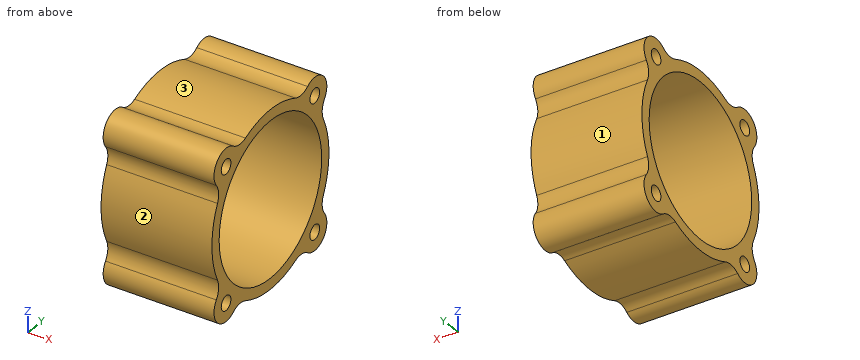
```python
from build123d import *

# Parameters (mm, degrees)
SKETCH_1_R      = 21.25
SKETCH_1_R_2    = 2
EXTRUDE_1_DEPTH = 15.2


with BuildPart() as part:
    # 草图1 → 凸台-拉伸1 (new body, symmetric)
    with BuildSketch(Plane(origin=(0, 0, 0), x_dir=(0, 0, -1), z_dir=(1, 0, 0))):
        with BuildLine():
            ThreePointArc((-15.431825442, 22.419634577), (-21.920310245, 21.920310245), (-22.419634577, 15.431825442))
            ThreePointArc((-22.419634577, 15.431825442), (-21.477282941, 12.955720303), (-21.932357291, 10.345733597))
            ThreePointArc((-21.932357291, 10.345733597), (-24.25, 0), (-21.932357291, -10.345733597))
            ThreePointArc((-21.932357291, -10.345733597), (-21.477282941, -12.955720303), (-22.419634577, -15.431825442))
            ThreePointArc((-22.419634577, -15.431825442), (-21.920310245, -21.920310245), (-15.431825442, -22.419634577))
            ThreePointArc((-15.431825442, -22.419634577), (-12.955720303, -21.477282941), (-10.345733597, -21.932357291))
            ThreePointArc((-10.345733597, -21.932357291), (0, -24.25), (10.345733597, -21.932357291))
            ThreePointArc((10.345733597, -21.932357291), (12.955720303, -21.477282941), (15.431825442, -22.419634577))
            ThreePointArc((15.431825442, -22.419634577), (21.920310245, -21.920310245), (22.419634577, -15.431825442))
            ThreePointArc((22.419634577, -15.431825442), (21.477282941, -12.955720303), (21.932357291, -10.345733597))
            ThreePointArc((21.932357291, -10.345733597), (24.25, 0), (21.932357291, 10.345733597))
            ThreePointArc((21.932357291, 10.345733597), (21.477282941, 12.955720303), (22.419634577, 15.431825442))
            ThreePointArc((22.419634577, 15.431825442), (21.920310245, 21.920310245), (15.431825442, 22.419634577))
            ThreePointArc((15.431825442, 22.419634577), (12.955720303, 21.477282941), (10.345733597, 21.932357291))
            ThreePointArc((10.345733597, 21.932357291), (0, 24.25), (-10.345733597, 21.932357291))
            ThreePointArc((-10.345733597, 21.932357291), (-12.955720303, 21.477282941), (-15.431825442, 22.419634577))
        make_face()
        Circle(SKETCH_1_R, mode=Mode.SUBTRACT)
        with Locations((-18.384776339, 18.384776339)):
            Circle(SKETCH_1_R_2, mode=Mode.SUBTRACT)
        with Locations((18.384776339, 18.384776339)):
            Circle(SKETCH_1_R_2, mode=Mode.SUBTRACT)
        with Locations((18.384776339, -18.384776339)):
            Circle(SKETCH_1_R_2, mode=Mode.SUBTRACT)
        with Locations((-18.384776339, -18.384776339)):
            Circle(SKETCH_1_R_2, mode=Mode.SUBTRACT)
    extrude(amount=EXTRUDE_1_DEPTH, both=True)


solid = part.part
```
The listing builds one solid part. Answer for the finished solid, in the listing's coordinates (mm). Face numbers are marked on the shaded views. Coordinates: 2 decimals unless noted, no trailing zeros. Loops run counter-clockwise (first coordinate to the right, second up) from the corner with the lowest first, then second, coordinate; pieces in that order, holes last. Notation, with made-up numbers: M 83,30 L 141,30 A23 cw 141,49 Z; hole C 23,-4 d9. An arc over 180 degrees is marked long. Answer as CSV lines item,"result". Start each with the question number.
(1) Given pin 1 (8 mm diameter, centred on x = -7.5, z = 14, fed in from -Y); pin 2 (3 mm diameter, centred on x = 1, z = -9, fed in from +Y); pin 3 (6 mm diameter, centred on x = 4.5, z = -4, fed in from -Y), each flat-ended and moving along its own axis, determine where each tip first touches the part or whether it passes through.
(2) The mould has two halves that part along Y. Classify the marked faces 1, 2 and 3: pulls with the +Y half, pulls with the -Y half, needs draft (parallel to the pull), parting line crosses it, or undercut.
(3) Find the intervals of material crossed by L1, parallel to Y at x = 8, z = 18; L2, parallel to Y at x = -12, z = 19.5; L3, parallel to Y at x = 4, z = 7, in increasing order. Write a range as [from, to].
(4) The part is cut by section A-A (z = 0). Give the vertices of the cut face in (x, y), and give its area (3 significant figures).
(5) The part is cut by section C-C (x = 13). Give the vertices of the cut face in (y, z).
Determined:
1,pin 1,"y = -23.37"
1,pin 2,"y = 23.06"
1,pin 3,"y = -24.23"
2,face 1,"pulls with the +Y half"
2,face 2,"pulls with the -Y half"
2,face 3,"undercut"
3,L1,"[-23.37, -20.35], [-16.42, -11.29], [11.29, 16.42], [20.35, 23.37]"
3,L2,"[-23.26, -20.04], [-16.72, -8.44], [8.44, 16.72], [20.04, 23.26]"
3,L3,"[-23.22, -20.06], [20.06, 23.22]"
4,outline,"M -15.2,-24.25 L 15.2,-24.25 L 15.2,-21.25 L -15.2,-21.25 Z; M -15.2,21.25 L 15.2,21.25 L 15.2,24.25 L -15.2,24.25 Z"
4,area,"182 mm2"
5,outline,"M -22.42,-15.43 A5 ccw -15.43,-22.42 A5 cw -10.35,-21.93 A24.25 ccw 10.35,-21.93 A5 cw 15.43,-22.42 A5 ccw 22.42,-15.43 A5 cw 21.93,-10.35 A24.25 ccw 21.93,10.35 A5 cw 22.42,15.43 A5 ccw 15.43,22.42 A5 cw 10.35,21.93 A24.25 ccw -10.35,21.93 A5 cw -15.43,22.42 A5 ccw -22.42,15.43 A5 cw -21.93,10.35 A24.25 ccw -21.93,-10.35 A5 cw Z; hole C 0,0 d42.5; hole C -18.38,-18.38 d4; hole C -18.38,18.38 d4; hole C 18.38,-18.38 d4; hole C 18.38,18.38 d4"
